Read the model definition and answer for the solid it produces. Units are mm, in the model's axes. A direction names the side the tool comes from. Give positions to 0.01 mm unless a question says otherwise; leave off trailing zeros. Order: outer loops, then holes, each group sorted by start corner. A loop starts at its lowest first (then second) coordinate and runs counter-clockwise, first axis right, second up. Notation, with made-up numbers: (84.25, -1) - (124.25, -1) arc R22 cw to (124.25, 17) - close; hole circle Ø6 at (-34.5, -32.5). An arc over 180 degrees is marked (long way). Write item = value, one per line.
```python
from build123d import *

# Parameters (mm, degrees)
F5_DEPTH  = 5
F6_R      = 4
F7_R      = 3.5
F8_DEPTH  = 22
F10_D     = 8
F10_DEPTH = 480
F10_TIP   = 2.4034424761


with BuildPart() as f1:
    # F0 (on Front) → F1 (revolve)
    with BuildSketch(Plane.XZ):
        with BuildLine():
            Line((0, -155.457497781), (0, 374.542502219))
            Line((0, 374.542502219), (-22, 374.542502219))
            Line((-22, 374.542502219), (-22, -25.457497781))
            Line((-22, -25.457497781), (-14.5, -25.457497781))
            ThreePointArc((-14.5, -25.457497781), (-13.0857864376, -26.0432842186), (-12.5, -27.457497781))
            Line((-12.5, -27.457497781), (-12.5, -54.457497781))
            Line((-12.5, -54.457497781), (-11, -54.457497781))
            Line((-11, -54.457497781), (-11, -56.457497781))
            Line((-11, -56.457497781), (-12.5, -56.457497781))
            Line((-12.5, -56.457497781), (-12.5, -135.457497781))
            Line((-12.5, -135.457497781), (-12, -135.457497781))
            ThreePointArc((-12, -135.457497781), (-10.5857864376, -136.0432842186), (-10, -137.457497781))
            Line((-10, -137.457497781), (-10, -155.457497781))
            Line((-10, -155.457497781), (0, -155.457497781))
        make_face()
    revolve(axis=Axis((0, 0, 132.3210597038), (0, 0, -1)))

    # F4 (on offset) → F5 (cut)
    with BuildSketch(Plane.XZ.offset(22)):
        with BuildLine():
            Line((6, 111.542502219), (6, 643.542502219))
            Line((6, 643.542502219), (-6, 643.542502219))
            Line((-6, 643.542502219), (-6, 111.542502219))
            ThreePointArc((-6, 111.542502219), (0, 105.542502219), (6, 111.542502219))
        make_face()
    extrude(amount=-F5_DEPTH, mode=Mode.SUBTRACT)

    # F6
    f6_edges = [f1.edges().sort_by_distance(p)[0] for p in [
        (10, 0, -155.457498),
    ]]
    fillet(f6_edges, radius=F6_R)

    # F7 (on offset) → F8 (cut)
    with BuildSketch(Plane.XZ.offset(22)):
        with Locations((0, -100.457497781)):
            Circle(F7_R)
    extrude(amount=-F8_DEPTH, mode=Mode.SUBTRACT)

    # F10
    with Locations(Plane.XY.offset(374.542502219)):
        with Locations((0, 0)):
            Hole(F10_D / 2, depth=F10_DEPTH)
            with Locations((0, 0, -(F10_DEPTH + F10_TIP / 2))):  # 118° drill point
                Cone(0, F10_D / 2, F10_TIP, mode=Mode.SUBTRACT)


solid = f1.part
```
1. Section B-B (z = 94) is taken. Determine the outline of the cut face in (x, y), and give its area (3 significant figures).
Recorded:
outline = circle Ø44 at (0, 0); hole circle Ø8 at (0, 0)
area = 1,470 mm^2
2. Section A-A (z = 170.5) is taken. Determine the outline of the cut face in (x, y), and give its area (3 significant figures).
Recorded:
outline = (-6, -21.17) - (-6, -17) - (6, -17) - (6, -21.17) arc R22 ccw (long way) to start; hole circle Ø8 at (0, 0)
area = 1,410 mm^2
3. Section C-C (z = -61.5) is taken. Determine the outline of the cut face in (x, y).
Recorded:
outline = circle Ø25 at (0, 0); hole circle Ø8 at (0, 0)
4. Flat-ended cylindrical pins translate along their axes: pin 1 (8 mm diameter, centred on y = 2.5, z = 254.5, fed in from +X); pin 2 (4 mm diameter, centred on y = 13, z = 203.5, fed in from +X); pin 3 (3.5 mm diameter, centred on y = -19.5, z = 273.5, fed in from +X); pin 4 (12 mm diameter, centred on x = 17, z = 199.5, fed in from -Y). Find the tip coordinate at first contact, or state that the pin passes through.
Recorded:
pin_1 = 22
pin_2 = 19.05
pin_3 = 13
pin_4 = -19.05
5. Determine the mould class of faces 5 (the face through (2.38, -10.74, -55.47)), 6 (the face through (0, 0, -155.457)), 7 (the face through (5, 1, 374.543)) for opening direction Z: +Z half, -Z half, draft (parallel to the pull), parting line (faces both ways), or undercut.
Recorded:
face_5 = undercut
face_6 = -Z half
face_7 = +Z half
6. Straight lines are drawn through the part: L1, parallel to Z at x = -2.5, y = 11.5; L2, parallel to X at y = 0, z = -3; L3, parallel to Z at x = 0, y = -5. For each, find the intervals that lie inside material, in ascending order. Write a range as [from, to].
Recorded:
L1 = [-135.47, -56.46], [-54.46, 374.54]
L2 = [-22, -4], [4, 22]
L3 = [-155.46, -103.96], [-96.96, 374.54]
7. For faces 1 (the face through (5, -10, -56.457)), 2 (the face through (-11.923, 3.755, -41.146)), 3 (the face through (-11.83, 18.55, 171.74)), 4 (the face through (0, -17, 242)), determine the directions among +Z, -Z, +X, -X, +Y, -Y from which every point of the face is accessible in a straight line to the end or side of a thin tool.
Recorded:
face_1 = none
face_2 = -Z
face_3 = +Z, -Z
face_4 = +Z, -Y
